from build123d import *

# Parameters (mm, degrees)
F0_W     = 30.4800020866
F0_H     = 16.8474918601
F0_H_2   = 38.1
F1_DEPTH = 33.782
F2_R     = 5.08


with BuildPart() as f1:
    # F0 (on Right) → F1 (new body)
    with BuildSketch(Plane.YZ):
        Polygon((35.8352853537, 66.4744316269), (-65.7647146463, 66.4744316269), (-65.7647146463, 28.3744316269), (-21.2170266578, 28.3744316269), (-21.2170266578, 45.221923487), (9.2629754288, 45.221923487), (9.2629754288, 28.3744316269), (35.8352853537, 28.3744316269), align=None)
        with Locations((-5.9770256145, 36.798177557)):
            Rectangle(F0_W, F0_H)
        with Locations((-5.9770256145, 9.3244316269)):
            Rectangle(F0_W, F0_H_2)
    extrude(amount=F1_DEPTH)

    # F2
    f2_edges = [f1.edges().sort_by_distance(p)[0] for p in [
        (0, -14.964715, 66.474432),
    ]]
    fillet(f2_edges, radius=F2_R)

    # F5: sweep along a path in F4
    with BuildLine(Plane.XZ.offset(65.7647146463)) as f5_path:
        Line((33.782, 42.0884639025), (60.0511431694, 42.0884639025))
        ThreePointArc((60.0511431694, 42.0884639025), (70.6826462574, 44.8201545239), (78.680468738, 52.3385205118))
        Line((78.680468738, 52.3385205118), (105.8331268172, 95.1905814836))
    # F3 (on face) → F5 (sweep)
    with BuildSketch(Plane.YZ.offset(33.782)):
        with BuildLine():
            Line((-65.7647146463, 33.2616948167), (-65.7647146463, 51.53828034))
            ThreePointArc((-65.7647146463, 51.53828034), (-74.903007408, 42.3999875784), (-65.7647146463, 33.2616948167))
        make_face()
        with BuildLine():
            ThreePointArc((-65.7647146463, 33.2616948167), (-59.3029658661, 35.9382387982), (-56.6264218847, 42.3999875784))
            ThreePointArc((-56.6264218847, 42.3999875784), (-59.3029658661, 48.8617363586), (-65.7647146463, 51.53828034))
            Line((-65.7647146463, 51.53828034), (-65.7647146463, 33.2616948167))
        make_face()
    sweep(path=f5_path.line)


solid = f1.part
Can you work these out from the model? Positions are in its coordinate system, mm. A direction names the side the tool comes from. Give positions to 0.01 mm unless a question says otherwise; leave off trailing zeros. Loops run counter-clockwise (first coordinate to the right, second up) from the corner with the lowest first, then second, coordinate; pieces in that order, holes last. Notation, with made-up numbers: M -3.5,-31.5 L 11.5,-31.5 A33 cw 11.5,7.5 Z; hole C 16,27 d4. An arc over 180 degrees is marked long. One line per item, written item: value. Start each with the question number.
1) On a 3-axis mill with a long thin cutter (end or side, diameter ignored), from which of +Z, -Z, +X, -X, +Y, -Y can I reach the whole of each face in a straight line? I mean faces 1 (the face through (17, 9.263, 9)), 2 (the face through (17, -44, 28.374)), 3 (the face through (17, -65.765, 48)), 4 (the face through (0, -16, 34)), 5 (the face through (17, 35.835, 47)). Say none if no direction works.
2) I'm going to push flat-ended pins straight in: pin 1 (8 mm diameter, centred on x = 21.5, y = 19, fed in from -Z); pin 2 (1.5 mm diameter, centred on y = -12.5, z = 53.5, fed in from +X); pin 3 (10 mm diameter, centred on x = 11.5, z = 49.5, fed in from -Y). Where does each tip first touch, or does it pass through?
3) If we section it at D-D, the plane y = 25.5: Write out the boundary of the cut face in (x, z).
4) If we section it at A-A, the plane y = 1.5: Write out the boundary of the cut face in (x, z).
5) If I drill on line 1 (Z direction, x = 20.5, y = -40.5); line 2 (Z direction, x = 27.5, y = -10.5); line 3 (X direction, y = -26, z = 51.5), over which ranges is the centre line in solid material (lowest first)? Write a range as [from, to].
6) If we section it at C-C, the plane x = 39.5: Write out the boundary of the cut face in (y, z).
7) If we section it at B-B, the plane z = 31: Write out the boundary of the cut face in (x, y), and give its area (3 significant figures).
Completed:
1. face 1: -Z, +X, -X, +Y
1. face 2: -Z, +X, -X, -Y
1. face 3: +Z, -Z, -X, -Y
1. face 4: +Z, -Z, -X, +Y, -Y
1. face 5: +Z, -Z, +X, -X, +Y
2. pin 1: stops at z = 28.37
2. pin 2: stops at x = 33.78
2. pin 3: stops at y = -65.76
3. outline: M 0,28.37 L 33.78,28.37 L 33.78,66.47 L 5.08,66.47 A5.08 ccw 0,61.39 Z
4. outline: M 0,-9.73 L 33.78,-9.73 L 33.78,66.47 L 5.08,66.47 A5.08 ccw 0,61.39 Z
5. line 1: z = [28.37, 66.47]
5. line 2: z = [-9.73, 66.47]
5. line 3: x = [0, 33.78]
6. outline: C -65.76,42.4 d18.28
7. outline: M 0,-65.76 L 33.78,-65.76 L 33.78,35.84 L 0,35.84 Z
7. area: 3,430 mm^2
